Autodesk Inventor part; units mm, degrees
ref_plane "YZ Plane" through (0, 0, 0) normal (1, 0, 0) x (0, 1, 0)
ref_plane "XZ Plane" through (0, 0, 0) normal (0, 1, 0) x (-1, 0, 0)
ref_plane "XY Plane" through (0, 0, 0) normal (0, 0, 1) x (1, 0, 0)
sketch "Sketch1" plane through (0, 0, 0) normal (0, 1, 0) x (-1, 0, 0)
  line L0 (0, 0) -> (-76.2, 0)
  line L1 (-76.2, 0) -> (-76.2, -50.8)
  line L2 (-76.2, -50.8) -> (0, -50.8)
  line L3 (0, -50.8) -> (0, 0)
  dimension "d0" = 76.2
  dimension "d1" = 50.8
extrude "Extrusion1" add sketch "Sketch1" along normal blind 12.7
chamfer "Chamfer1" distance 12.7 distance2 3.175 1 edges at (38.1, 0, -50.8) measured on face at (50.8, 4.2333, -50.8)
chamfer "Chamfer2" distance 12.7 distance2 3.175 1 edges at (38.1, 0, 0) measured on face at (25.4, 4.2333, 0)
chamfer "Chamfer3" distance 12.7 distance2 3.175 1 edges at (76.2, 0, -25.4) measured on face at (76.2, 8.4663, -32.8085)
chamfer "Chamfer4" distance 12.7 distance2 3.175 1 edges at (0, 0, -25.4) measured on face at (0, 8.4663, -17.9915)
sketch "Sketch2" plane through (0, 12.7, 0) normal (0, 1, 0) x (1, 0, 0)
  line L0 (0, 50.8) -> (3.175, 47.625)
  line L1 (0, 0) -> (76.2, 0)
  line L2 (0, 50.8) -> (76.2, 50.8)
  line L3 (76.2, 50.8) -> (76.2, 0)
  line L4 (76.2, 0) -> (0, 0)
  line L5 (0, 0) -> (0, 50.8)
extrude "Extrusion2" add sketch "Sketch2" along normal blind 25.4
chamfer "Chamfer5" distance 5.08 distance2 25.4 1 edges at (38.1, 38.1, 0) measured on face at (25.4, 38.1, -33.8667)
chamfer "Chamfer6" distance 5.08 distance2 25.4 1 edges at (38.1, 38.1, -50.8) measured on face at (50.8, 38.1, -20.32)
chamfer "Chamfer7" distance 38.1 distance2 25.4 1 edges at (0, 38.1, -25.4) measured on face at (50.8, 38.1, -18.6267)
chamfer "Chamfer8" distance 38.1 distance2 25.4 1 edges at (76.2, 38.1, -25.4) measured on face at (50.8, 38.1, -32.1733)
sketch "Sketch6" plane through (3.175, 0, -3.175) normal (0, -0.2425, 0.9701) x (1, 0, 0)
  line L0 (0, 0) -> (69.85, 0)
  line L1 (0, 0) -> (15.24, 0)
  line L2 (15.24, 0) -> (24.13, 0)
  line L3 (69.85, 0) -> (69.85, -10.7807)
  line L4 (69.85, 0) -> (54.61, 0)
  line L5 (54.61, 0) -> (45.72, 0)
  line L6 (24.13, 0) -> (19.685, -7.699)
  line L7 (19.685, -7.699) -> (10.795, -7.699)
  line L8 (10.795, -7.699) -> (6.35, 0)
  line L9 (6.35, 0) -> (10.795, 7.699)
  line L10 (10.795, 7.699) -> (19.685, 7.699)
  line L11 (19.685, 7.699) -> (24.13, 0)
  line L12 (45.72, 0) -> (50.165, 7.699)
  line L13 (50.165, 7.699) -> (59.055, 7.699)
  line L14 (59.055, 7.699) -> (63.5, 0)
  line L15 (63.5, 0) -> (59.055, -7.699)
  line L16 (59.055, -7.699) -> (50.165, -7.699)
  line L17 (50.165, -7.699) -> (45.72, 0)
  point P0 (-3.175, 0.7701)
  dimension "d34" = 15.24
  dimension "d35" = 8.89
  dimension "d36" = 15.24
  dimension "d37" = 8.89
extrude "Extrusion3" cut sketch "Sketch6" against normal blind 7.62 contours L9 L10 L11 L0 | L0 L6 L7 L8
sketch "Sketch7" plane through (0, 12.7, 0) normal (0, -0.2425, 0.9701) x (1, 0, 0)
  line L0 (27.305, -13.0909) -> (73.025, -13.0909)
  line L1 (73.025, -13.0909) -> (57.785, -13.0909)
  line L2 (57.785, -13.0909) -> (48.895, -13.0909)
  line L3 (48.895, -13.0909) -> (53.34, -5.3919)
  line L4 (53.34, -5.3919) -> (62.23, -5.3919)
  line L5 (62.23, -5.3919) -> (66.675, -13.0909)
  line L6 (66.675, -13.0909) -> (62.23, -20.7898)
  line L7 (62.23, -20.7898) -> (53.34, -20.7898)
  line L8 (53.34, -20.7898) -> (48.895, -13.0909)
  point P0 (0, -12.3208)
  dimension "d40" = 15.24
  dimension "d41" = 8.89
extrude "Extrusion4" cut sketch "Sketch7" against normal blind 7.62
sketch "Sketch8" plane through (73.025, 0, -47.625) normal (0, -0.2425, -0.9701) x (-1, 0, 0)
  line L0 (69.85, 0) -> (69.85, -10.7807)
  line L1 (69.85, 0) -> (54.61, 0)
  line L2 (0, 0) -> (69.85, 0)
  line L3 (54.61, 0) -> (45.72, 0)
  line L4 (45.72, 0) -> (50.165, 7.699)
  line L5 (50.165, 7.699) -> (59.055, 7.699)
  line L6 (59.055, 7.699) -> (63.5, 0)
  line L7 (63.5, 0) -> (59.055, -7.699)
  line L8 (59.055, -7.699) -> (50.165, -7.699)
  line L9 (50.165, -7.699) -> (45.72, 0)
  point P0 (73.025, -11.5508)
  dimension "d44" = 15.24
  dimension "d45" = 8.89
extrude "Extrusion5" cut sketch "Sketch8" against normal blind 7.62
properties part number "tesla v1"
Work out the finished part from the listing and answer in its coordinate system (mm). A direction names the side the tool comes from. Coordinates: 2 decimals unless noted, no trailing zeros. Loops run counter-clockwise (first coordinate to the right, second up) from the corner with the lowest first, then second, coordinate; pieces in that order, holes last. Notation, with made-up numbers: M -32,53.5 L -9,53.5 A34 cw -9,84.5 Z; hole C 19.25,70 d7. An arc over 180 degrees is marked long. Answer in a Markdown table with one row per item. Add a question column.
1. Find section B-B, the plane y = 6.5. Write down the section's boundary in (x, z), then the cut area to 3 significant figures.
2. Flat-ended cylindrical pins translate along their axes: P1, Ø5, axis at x = 14, y = 19, coming from the +Z side; P2, Ø5, axis at x = 59, z = -12, coming from the +Y side; P3, Ø5, axis at x = 24.5, y = 6.5, coming from the -Z side. Find the tip coordinate at first contact, or state that the pin passes through.
3. The mould has two halves that part along Z. Classify faces 4 (the flat face through (38.633, 7.672, -1.257)), 5 (the flat face through (37.57, 22.4, -48.86)), 6 (the flat face through (9.823, 0.822, -42.211)), 7 (the flat face through (25.05, 4.7, -5.87)): pulls with the +Z half, pulls with the -Z half, needs draft (parallel to the pull), parting line crosses it, or undercut.
4. Consider L1, parallel to X at y = 6.5, z = -7; L2, parallel to Z at x = 45, y = 7.5; L3, parallel to Y at x = 32.5, z = -12. Determine where each line is inside the solid, lowest interval first.
5. A tool of negligible diameter and unlimited length cuts with its end or side. For faces 1 (the flat face through (9.838, 0.796, -8.595)), 2 (the flat face through (18.78, 25.22, -25.04)), 3 (the flat face through (18.48, 8.38, -45.85)), from which of +Z, -Z, +X, -X, +Y, -Y can it reach the whole face along a straight path? Write none if from no direction.
Reported:
| question | item | result |
|---|---|---|
| 1 | outline | M 1.55,-49.25 L 13.39,-49.25 L 12.29,-41.39 L 24.54,-41.39 L 23.44,-49.25 L 74.65,-49.25 L 74.65,-1.55 L 62.81,-1.55 L 63.91,-9.41 L 51.66,-9.41 L 52.76,-1.55 L 23.44,-1.55 L 24.54,-9.41 L 12.29,-9.41 L 13.39,-1.55 L 1.55,-1.55 Z |
| 1 | area | 3,220 mm^2 |
| 2 | P1 | stops at z = -0.76 |
| 2 | P2 | stops at y = 25.83 |
| 2 | P3 | stops at z = -49.88 |
| 3 | face 4 | pulls with the +Z half |
| 3 | face 5 | pulls with the -Z half |
| 3 | face 6 | undercut |
| 3 | face 7 | undercut |
| 4 | L1 | x = 1.55 to 12.63, 24.2 to 52, 63.57 to 74.65 |
| 4 | L2 | z = -49.5 to -1.3 |
| 4 | L3 | y = 0 to 34.37 |
| 5 | face 1 | none |
| 5 | face 2 | +Z, -Z, -X, +Y |
| 5 | face 3 | -Y |
